```python
from build123d import *

# Parameters (mm, degrees)
BOSS_EXTRUDE1_DEPTH     = 4
SKETCH2_W               = 20
SKETCH2_H               = 25
CUT_EXTRUDE1_DEPTH      = 2
CUT_EXTRUDE2_DEPTH      = 78.013058248
CUT_EXTRUDE2_DEPTH_BACK = 78.013058248
CUT_EXTRUDE3_DEPTH      = 78.013058248
LPATTERN1_COUNT         = 26
LPATTERN1_PITCH         = 1.0025
CUT_EXTRUDE4_DEPTH      = 78.013058248
CUT_EXTRUDE5_DEPTH      = 78.013058248
FILLET1_R               = 10
FILLET2_R               = 2
FILLET3_R               = 1
FILLET4_R               = 0.5
SKETCH9_R               = 1.5
SKETCH9_R_2             = 1.652612025
CUT_EXTRUDE6_DEPTH      = 77.755921087


with BuildPart() as part:
    # Sketch1 → Boss-Extrude1 (new, symmetric)
    with BuildSketch(Plane.XY):
        Polygon((0, 0), (-20, 29.933259094), (-20, 60.063259094), (-21.435566599, 72.983752449), (-16.466146078, 73.535893449), (-14.000284373, 51.342461401), (-14.000284373, 49.942461401), (0, 39.956155609), align=None)
    extrude(amount=BOSS_EXTRUDE1_DEPTH, both=True)

    # Sketch2 → Cut-Extrude1 (cut, symmetric)
    with BuildSketch(Plane.XY):
        with Locations((-24.000284373, 62.442461401)):
            Rectangle(SKETCH2_W, SKETCH2_H)
    extrude(amount=CUT_EXTRUDE1_DEPTH, both=True, mode=Mode.SUBTRACT)

    # Sketch3 → Cut-Extrude2 (cut, two sides: drawn at the far end of the back side and taken through both)
    with BuildSketch(Plane.XY.offset(4).offset(-CUT_EXTRUDE2_DEPTH_BACK)):
        with BuildLine():
            Line((91.496624596, 102.578624056), (0, 33.956155609))
            ThreePointArc((0, 33.956155609), (-2, 29.956155609), (0, 25.956155609))
            Line((0, 25.956155609), (91.496624596, -42.666312838))
            Line((91.496624596, -42.666312838), (320.238186086, -42.666312838))
            Line((320.238186086, -42.666312838), (320.238186086, 102.578624056))
            Line((320.238186086, 102.578624056), (91.496624596, 102.578624056))
        make_face()
    extrude(amount=CUT_EXTRUDE2_DEPTH + CUT_EXTRUDE2_DEPTH_BACK, mode=Mode.SUBTRACT)

    # Sketch4 → Cut-Extrude3 (cut, symmetric)
    with BuildSketch(Plane.XY.offset(4)):
        Polygon((51.965078117, 129.886311843), (0, 25.956155609), (-0.5, 24.956155609), (0, 24.956155609), (116.197447126, 24.956155609), (314.404638126, 146.287504856), (250.172269117, 251.21766109), align=None)
    cut_extrude3 = extrude(amount=CUT_EXTRUDE3_DEPTH, both=True, mode=Mode.SUBTRACT)

    # LPattern1: Cut-Extrude3 ×26
    with Locations(*[(0, -i * LPATTERN1_PITCH, 0) for i in range(1, LPATTERN1_COUNT)]):
        add(cut_extrude3, mode=Mode.SUBTRACT)

    # Sketch5 → Cut-Extrude4 (cut, through all)
    with BuildSketch(Plane.XY.offset(4)):
        with BuildLine():
            Line((-20, 44.933259094), (-20, 29.933259094))
            Line((-20, 29.933259094), (-6.933333333, 10.376863153))
            ThreePointArc((-6.933333333, 10.376863153), (-12.465928354, 28.033466151), (-20, 44.933259094))
        make_face()
    extrude(amount=-CUT_EXTRUDE4_DEPTH, mode=Mode.SUBTRACT)

    # Sketch6 → Cut-Extrude5 (cut, through all)
    with BuildSketch(Plane.XY.offset(4)):
        with BuildLine():
            Line((-14.004117633, 45.031887994), (-5, 38.609313304))
            Line((-5, 38.609313304), (-5, 17.671887994))
            ThreePointArc((-5, 17.671887994), (-9.031897039, 29.700512127), (-14.004117633, 41.371887994))
            Line((-14.004117633, 41.371887994), (-14.004117633, 45.031887994))
        make_face()
    extrude(amount=-CUT_EXTRUDE5_DEPTH, mode=Mode.SUBTRACT)

    # Fillet1
    fillet1_edges = [part.edges().sort_by_distance(p)[0] for p in [
        (0, 39.956155609, 0),
        (-20, 44.933259094, 0),
        (-6.933333333, 10.376863153, 0),
    ]]
    fillet(fillet1_edges, radius=FILLET1_R)

    # Fillet2
    fillet2_edges = [part.edges().sort_by_distance(p)[0] for p in [
        (-21.435566599, 72.983752449, 3),
        (-16.466146078, 73.535893449, 3),
        (-14.000284373, 49.942461401, 3),
        (-21.435566599, 72.983752449, -3),
        (-16.466146078, 73.535893449, -3),
        (-14.000284373, 49.942461401, -3),
    ]]
    fillet(fillet2_edges, radius=FILLET2_R)

    # Fillet3
    fillet3_edges = [part.edges().sort_by_distance(p)[0] for p in [
        (-14.004117633, 41.371887994, 0),
        (-14.004117633, 45.031887994, 0),
        (-5, 38.609313304, 0),
    ]]
    fillet(fillet3_edges, radius=FILLET3_R)

    # Fillet4
    fillet4_edges = [part.edges().sort_by_distance(p)[0] for p in [
        (-5, 17.671887994, 0),
    ]]
    fillet(fillet4_edges, radius=FILLET4_R)

    # Sketch9 → Cut-Extrude6 (cut, through all)
    with BuildSketch(Plane.XY.offset(4)):
        with Locations((-18.416383851, 68.449423885)):
            Circle(SKETCH9_R)
        with Locations((-16.915664614, 54.942538908)):
            Circle(SKETCH9_R_2)
    extrude(amount=-CUT_EXTRUDE6_DEPTH, mode=Mode.SUBTRACT)


solid = part.part
```
For this review, take the finished solid that the model builds, in its own axes (mm). A direction names the side the tool comes from. Give positions to 0.01 mm unless a question says otherwise; leave off trailing zeros. Loops run counter-clockwise (first coordinate to the right, second up) from the corner with the lowest first, then second, coordinate; pieces in that order, holes last. Notation, with made-up numbers: M 69.25,11.5 L 101.25,11.5 A23 cw 101.25,47.5 Z; hole C 85.25,-30 d8. An arc over 180 degrees is marked long. One line per item, written item: value. Start each with the question number.
Q1. Add section C-C (z = -3). Count the separate pieces of the cut face and the enclosed holes in it, and give its area (3 significant figures).
Q2. Machinability: for faces 5 (the face through (-20, 52, 3)), 6 (the face through (-13.77, 50.04, -2.99)), 7 (the face through (-13.448, 43.986, -0.056)), 8 (the face through (-17, 49.942, 0)), which of the approach directions +Z, -Z, +X, -X, +Y, -Y give a long, thin tool a straight path to every point of the face, cutting with its end or side? Answer none if there is none.
Q3. Add section B-B (y = 36). Give the boundary of the cut face in (x, z), and give its area (3 significant figures).
Q4. For L1, parallel to Z at x = -16.5, y = 67.5; L2, parallel to X at y = 29.5, z = -1.5; L3, parallel to Y at x = -16.5, z = 2.5, list the stretches that pass through material, from the lowest coordinate up.
Q5. Add section A-A (x = -8.75). Give the boundary of the cut face in (y, z).
Q6. Add section D-D (y = 45.5). Give the boundary of the cut face in (x, z).
Q7. Clearance check with flat-ended pins moving along their axes: pin 1 Ø4 at (y, z) = (14.5, -3) entering from -X; pin 2 Ø2 at (x, y) = (-16.92, 54.94) entering from -Z. State where each tip first meets the part, or that it passes through.
Q8. Draft analysis for pull direction Z (two halves, no side actions). For faces 1 (the face through (-11, 32, 4)), 2 (the face through (-18, 62, -2)), 3 (the face through (-11, 32, -4)), 4 (the face through (-19.726, 45.002, -0.056)), state which applies: released by +Z, released by -Z, zero draft, split by the parting line, or undercut.
Reply:
1. separate pieces: 1
1. enclosed holes: 3
1. area: 489 mm²
2. face 5: +Z, -Z, -X, -Y
2. face 6: +Z, -Z, +X, +Y
2. face 7: +Z, -Z
2. face 8: +X, -X, +Y
3. outline: M -15.73,-4 L -11.58,-4 L -11.58,4 L -15.73,4 Z; M -5,-4 L -0.07,-4 L -0.07,4 L -5,4 Z
3. area: 72.6 mm²
4. L1: -4 to -2, 2 to 4
4. L2: -13.03 to -8.96, -5 to -1.98
4. L3: 37.73 to 53.34, 56.54 to 72.33
5. outline: M 17.01,-4 L 28.95,-4 L 28.95,4 L 17.01,4 Z; M 41.28,-4 L 46.2,-4 L 46.2,4 L 41.28,4 Z
6. outline: M -19.83,-4 L -7.77,-4 L -7.77,4 L -19.83,4 Z
7. pin 1: x = -8.6
7. pin 2: through
8. face 1: released by +Z
8. face 2: undercut
8. face 3: released by -Z
8. face 4: zero draft
